The model under review builds one solid part; all positions refer to its coordinate system, in mm. Face numbers are marked on the shaded views. Coordinates: 2 decimals unless noted, no trailing zeros. Loops run counter-clockwise (first coordinate to the right, second up) from the corner with the lowest first, then second, coordinate; pieces in that order, holes last. Notation, with made-up numbers: (19.5, -33) -> (40.5, -33) arc R28 cw to (40.5, -9) -> close; hole circle Ø11 at (68, -26). An arc over 180 degrees is marked (long way). One line per question, with ' | ' between items. Start each with the question number.
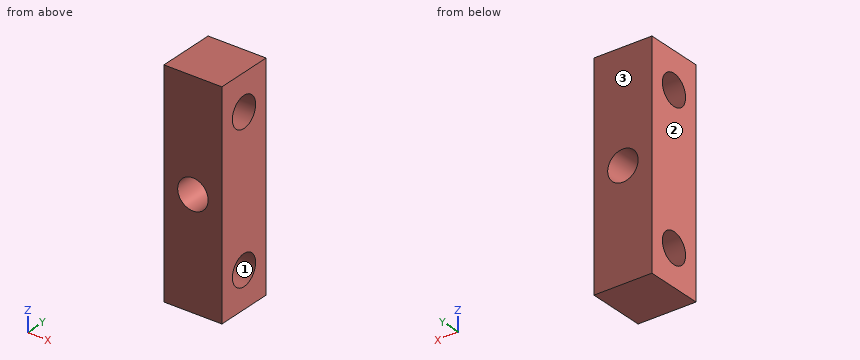
from build123d import *

# Parameters (mm, degrees)
SKETCH_2_W          = 8
SKETCH_2_H          = 8
EXTRUDE_1_DEPTH     = 30
SKETCH_3_R          = 2.1
CUT_EXTRUDE_1_DEPTH = 32.304951685
SKETCH_4_R          = 2.1
CUT_EXTRUDE_2_DEPTH = 32.304951685


with BuildPart() as part:
    # 草图2 → 凸台-拉伸1 (new body)
    with BuildSketch(Plane.XY):
        Rectangle(SKETCH_2_W, SKETCH_2_H)
    extrude(amount=EXTRUDE_1_DEPTH)

    # 草图3 → 切除-拉伸1 (cut, through all)
    with BuildSketch(Plane(origin=(0, 4, 0), x_dir=(1, 0, 0), z_dir=(0, 1, 0))):
        with Locations(Location((0, -15, 0), (0, 0, 270))):
            Circle(SKETCH_3_R)
    extrude(amount=-CUT_EXTRUDE_1_DEPTH, mode=Mode.SUBTRACT)

    # 草图4 → 切除-拉伸2 (cut, through all)
    with BuildSketch(Plane(origin=(4, 0, 0), x_dir=(0, 0, -1), z_dir=(1, 0, 0))):
        with Locations((-25, 0)):
            Circle(SKETCH_4_R)
        with Locations((-5, 0)):
            Circle(SKETCH_4_R)
    extrude(amount=-CUT_EXTRUDE_2_DEPTH, mode=Mode.SUBTRACT)


solid = part.part
1) Consider section B-B, the plane z = 25. Write out the cut boundary in (x, y), plus the area to 3 significant figures.
2) Consider section D-D, the plane x = -3. Write out the cut boundary in (y, z), plus the area to 3 significant figures.
3) Consider section C-C, the plane x = -1.5. Write out the cut boundary in (y, z).
4) Wall thickness on L1, parallel to X at y = 1.25, z = 15; L2, parallel to Z at x = 0.25, y = 1.75: over which ranges is each line inside the solid? List them lowest first.
5) Consider section A-A, the plane y = 0. Write out the cut boundary in (x, z), plus the area to 3 significant figures.
6) Mouldability with a two-part tool opening along Y and no side actions: class the marked faces 1, 2 and 3 as +Y half, -Y half, draft (parallel to the pull), parting line (faces both ways), or undercut.
7) Insertion check: pin 1 Ø4 at (y, z) = (0, 25) entering from +X. The pin has a flat end and moves straight along its axis. Give the tip position at first contact, or say it passes through.
Filled sheet:
1) outline: (-4, -4) -> (4, -4) -> (4, -2.1) -> (-4, -2.1) -> close; (-4, 2.1) -> (4, 2.1) -> (4, 4) -> (-4, 4) -> close | area: 30.4 mm^2
2) outline: (-4, 0) -> (4, 0) -> (4, 30) -> (-4, 30) -> close; hole circle Ø4.2 at (0, 5); hole circle Ø4.2 at (0, 25) | area: 212 mm^2
3) outline: (-4, 0) -> (4, 0) -> (4, 13.53) -> (-4, 13.53) -> close; (-4, 16.47) -> (4, 16.47) -> (4, 30) -> (-4, 30) -> close; hole circle Ø4.2 at (0, 5); hole circle Ø4.2 at (0, 25)
4) L1: -4 to -2.1, 2.1 to 4 | L2: 0 to 3.84, 6.16 to 12.91, 17.09 to 23.84, 26.16 to 30
5) outline: (-4, 0) -> (4, 0) -> (4, 2.9) -> (-4, 2.9) -> close; (-4, 7.1) -> (4, 7.1) -> (4, 22.9) -> (-4, 22.9) -> close; (-4, 27.1) -> (4, 27.1) -> (4, 30) -> (-4, 30) -> close; hole circle Ø4.2 at (0, 15) | area: 159 mm^2
6) face 1: undercut | face 2: draft | face 3: +Y half
7) pin 1: through
